Design review of the part shown in the three views and the two pictorial views. Dimensions are in mm from the part's minimum x, y and z. Give positions to 0.01 mm unless a question says otherwise; leave off trailing zeros. Order: outer loops, then holes, each group sorted by start corner. A loop starts at its lowest first (then second) coordinate and runs counter-clockwise, first axis right, second up.
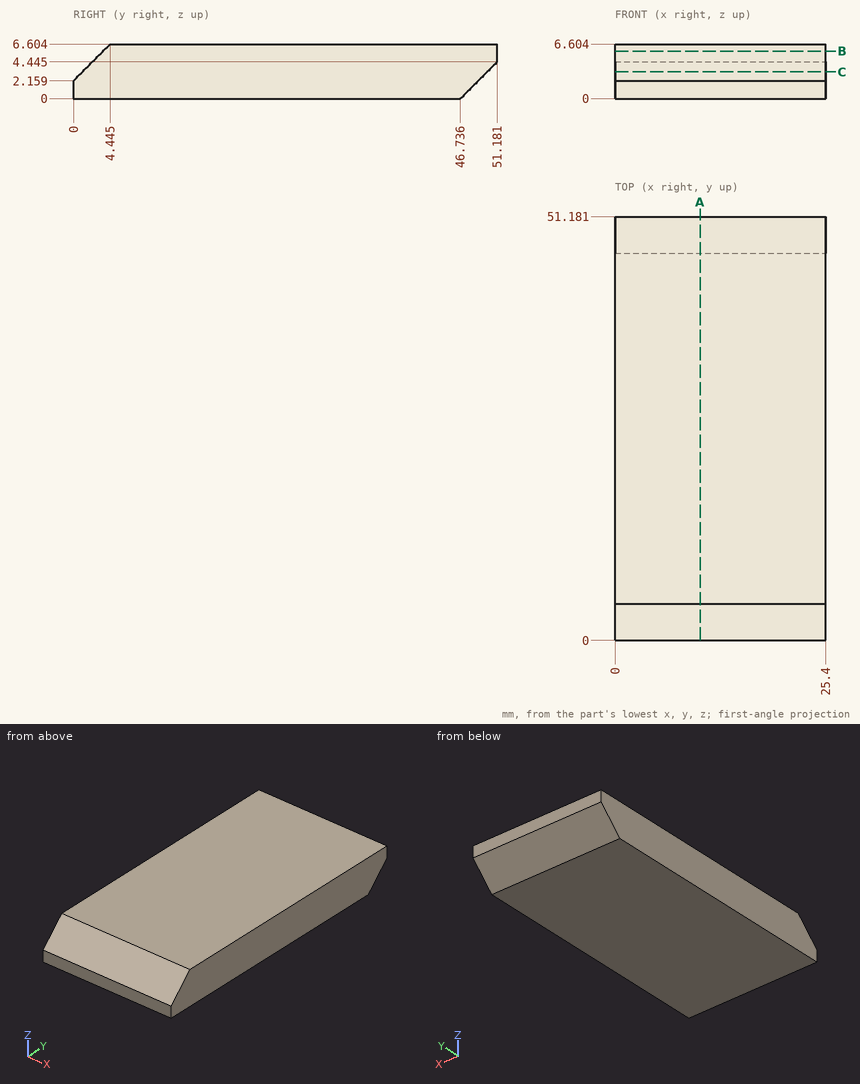
Item 1: Take a section at B-B (z = 5.75). Give the boundary of the cut face in (x, y).
Values found:
outline: (0, 3.59) - (25.4, 3.59) - (25.4, 51.18) - (0, 51.18) - close
Item 2: For line 1 (Y direction, x = 1.75, z = 5); line 2 (Y direction, x = 15, z = 3.25), list the stretches that pass through material, from the lowest coordinate up.
Values found:
line 1: y = 2.84 to 51.18
line 2: y = 1.09 to 49.99
Item 3: Take a section at A-A (x = 10.25). Give the boundary of the cut face in (y, z) (3 decimals).
Values found:
outline: (0, 0) - (46.736, 0) - (51.181, 4.445) - (51.181, 6.604) - (4.445, 6.604) - (0, 2.159) - close
Item 4: Take a section at C-C (z = 3.25). Give the boundary of the cut face in (x, y).
Values found:
outline: (0, 1.09) - (25.4, 1.09) - (25.4, 49.99) - (0, 49.99) - close
